Verification items for the finished model (mm, model axes). A direction names the side the tool comes from. Coordinates: 2 decimals unless noted, no trailing zeros. Order: outer loops, then holes, each group sorted by start corner. A loop starts at its lowest first (then second) coordinate and runs counter-clockwise, first axis right, second up. Notation, with made-up numbers: M 46.5,57.25 L 94.5,57.25 A36 cw 94.5,91.25 Z; hole C 86.25,51 d8. An arc over 180 degrees is marked long. Return JSON: item names as keys, results as strings. Group by question number.
1. Mould release check, pull along Z, two halves, no side actions. Record for faces 5 (the flat face through (12, -13, 11)), 6 (the flat face through (75, -6, 21)), 7 (the flat face through (75, -12, 25)): +Z half, -Z half, draft (parallel to the pull), parting line (faces both ways), or undercut.
2. Section check B-B, the plane z = 24. Record the cut outline in (x, y), plus the area to 3 significant figures.
3. Set-up check for faces 1 (the flat face through (68, -6, 22)), 2 (the flat face through (15, -7, 2)), 3 (the flat face through (9, -6, 3)), 4 (the cylindrical face through (80.479, -5.195, 25.487)): record each of +Z, -Z, +X, -X, +Y, -Y from which the full face is reachable in a straight line by a thin tool's end or side.
4. Section check C-C, the plane y = -13.5. Record the cut outline in (x, z), plus the area to 4 significant figures.
5. Gauge pin test, flat ends, axial feed: pin 1 (0.9 mm diameter, centred on y = -14, z = 9, fed in from +X); pin 2 (3.5 mm diameter, centred on x = 37.5, y = -8, fed in from -Z); pin 3 (0.9 mm diameter, centred on y = -6.5, z = 1, fed in from +X). Record the tip position at first contact, or that the pin passes through.
6. Section check D-D, the plane x = 21.5. Record the cut outline in (y, z), plus the area to 3 significant figures.
7. Material ranges on line 1 along X through (y, z) = (-10.5, 22); line 2 along Z through (x, y) = (81.3, -5); line 3 along Y through (x, z) = (10, 24.5), recorded low to high.
8. Section check A-A, the plane y = -5. Record the cut outline in (x, z).
```python
from build123d import *

# Parameters (mm, degrees)
PAD_DEPTH      = 12
PAD001_DEPTH   = 3
CYLINDER_R     = 1.5
CYLINDER_DEPTH = 3


with BuildPart() as part:
    # Sketch → Pad (new body)
    with BuildSketch(Plane.XZ):
        Polygon((82, 18), (82, 28), (79, 28), (79, 21), (71, 21), (71, 28), (0, 28), (0, 0), (15, 0), (15, 3), (3, 3), (3, 25), (68, 25), (68, 18), align=None)
    extrude(amount=PAD_DEPTH)

    # Sketch001 → Pad001 (join)
    with BuildSketch(Plane.XZ.offset(12)):
        Polygon((0, 28), (82, 28), (82, 18), (12, 18), (12, 3), (15, 3), (15, 0), (0, 0), align=None)
    extrude(amount=PAD001_DEPTH)

    # Cylinder → Cylinder (cut)
    with BuildSketch(Plane(origin=(79, -5, 24), x_dir=(0, 1, 0), z_dir=(1, 0, 0))):
        Circle(CYLINDER_R)
    extrude(amount=CYLINDER_DEPTH, mode=Mode.SUBTRACT)


solid = part.part
```
Answers follow:
{
 "1": {"face 5": "undercut", "face 6": "+Z half", "face 7": "draft"},
 "2": {"outline": "M 0,-15 L 82,-15 L 82,-6.5 L 79,-6.5 L 79,-12 L 71,-12 L 71,0 L 68,0 L 68,-12 L 3,-12 L 3,0 L 0,0 Z; M 79,-3.5 L 82,-3.5 L 82,0 L 79,0 Z", "area": "345 mm^2"},
 "3": {"face 1": "-Z, +Y", "face 2": "-Z, +X, +Y, -Y", "face 3": "+X, +Y", "face 4": "+X"},
 "4": {"outline": "M 0,0 L 15,0 L 15,3 L 12,3 L 12,18 L 82,18 L 82,28 L 0,28 Z", "area": "1,045 mm^2"},
 "5": {"pin 1": "x = 12", "pin 2": "z = 25", "pin 3": "x = 15"},
 "6": {"outline": "M -15,18 L -12,18 L -12,25 L 0,25 L 0,28 L -15,28 Z", "area": "66.0 mm^2"},
 "7": {"line 1": "0 to 3, 68 to 71, 79 to 82", "line 2": "18 to 22.5, 25.5 to 28", "line 3": "-15 to -12"},
 "8": {"outline": "M 0,0 L 15,0 L 15,3 L 3,3 L 3,25 L 68,25 L 68,18 L 82,18 L 82,22.5 L 79,22.5 L 79,21 L 71,21 L 71,28 L 0,28 Z; M 79,25.5 L 82,25.5 L 82,28 L 79,28 Z"}
}
